```python
from build123d import *

# Parameters (mm, degrees)
SKIZZE19_W = 1.85
SKIZZE19_H = 1
SKIZZE20_W = 1.85
SKIZZE20_H = 1
SKETCH1_W  = 14.101371306
SKETCH1_H  = 11.293421516


with BuildPart() as part:
    # Skizze1 → Rotation1 (revolve)
    with BuildSketch(Plane.XY, mode=Mode.PRIVATE) as rotation1_sk:
        Polygon((180, 19), (180, 0), (-180, 0), (-180, 19), (-79, 19), (-79, 27), (-74, 27), (-74, 19.001), (-44, 19.001), (-44, 19), align=None)
    revolve(rotation1_sk.sketch.rotate(Axis((180, 0, 0), (-1, 0, 0)), 90), axis=Axis((180, 0, 0), (-1, 0, 0)))

    # Skizze19 → Schnitt-Rotation1 (revolve, cut)
    with BuildSketch(Plane.XY, mode=Mode.PRIVATE) as schnitt_rotation1_sk:
        with Locations((171.825, 18.5)):
            Rectangle(SKIZZE19_W, SKIZZE19_H)
    revolve(schnitt_rotation1_sk.sketch.rotate(Axis((-88.99, 0, 0), (1, 0, 0)), 270), axis=Axis((-88.99, 0, 0), (1, 0, 0)), mode=Mode.SUBTRACT)

    # Skizze20 → Schnitt-Rotation2 (revolve, cut)
    with BuildSketch(Plane.XY, mode=Mode.PRIVATE) as schnitt_rotation2_sk:
        with Locations((-171.825, 18.5)):
            Rectangle(SKIZZE20_W, SKIZZE20_H)
    revolve(schnitt_rotation2_sk.sketch.rotate(Axis((-88.99, 0, 0), (1, 0, 0)), 270), axis=Axis((-88.99, 0, 0), (1, 0, 0)), mode=Mode.SUBTRACT)

    # Sketch1 → Cut-Revolve1 (revolve, cut)
    with BuildSketch(Plane.XY, mode=Mode.PRIVATE) as cut_revolve1_sk:
        with Locations((-76.280304753, 24.646710758)):
            Rectangle(SKETCH1_W, SKETCH1_H)
    revolve(cut_revolve1_sk.sketch.rotate(Axis((-191.164691911, 0, 0), (1, 0, 0)), 90), axis=Axis((-191.164691911, 0, 0), (1, 0, 0)), mode=Mode.SUBTRACT)


solid = part.part
```
The listing builds one solid part. Answer for the finished solid, in the listing's coordinates (mm). A direction names the side the tool comes from. Give positions to 0.01 mm unless a question says otherwise; leave off trailing zeros. Order: outer loops, then holes, each group sorted by start corner. A loop starts at its lowest first (then second) coordinate and runs counter-clockwise, first axis right, second up. Notation, with made-up numbers: (-16, 8.5) -> (0, 8.5) arc R21 cw to (0, 37.5) -> close; hole circle Ø6 at (-26.5, -37.75). An arc over 180 degrees is marked (long way). Answer as a JSON object with one key per item and string values. Group by question number.
Item 1: Flat-ended cylindrical pins translate along their axes: pin 1 (3 mm diameter, centred on x = -58, z = 12, fed in from +Y); pin 2 (12 mm diameter, centred on x = 71, z = 3, fed in from -Y); pin 3 (6 mm diameter, centred on x = 109, y = -11, fed in from -Z). Find the tip coordinate at first contact, or state that the pin passes through.
Item 2: Determine the mould class of faces 1 (the flat face through (180, 0, 0)), 2 (the flat face through (-180, 0, 0)), 3 (the flat face through (-170.9, -17, 7)) for opening direction X: pulls with the +X half, pulls with the -X half, needs draft (parallel to the pull), parting line crosses it, or undercut.
Item 3: Consider L1, parallel to X at y = -12.5, z = 13; L2, parallel to Y at x = -81.5, z = -0.5; L3, parallel to Z at x = 116.5, y = -1.5. Determine where each line is inside the solid, lowest interval first. Write a range as from..to.
Item 4: The part is cut by section B-B on x = -102. Write down the section's boundary in (y, z).
Item 5: A tool of negligible diameter and unlimited length cuts with its end or side. For faces 4 (the cylindrical face through (64.954, 18.548, 4.119)), 5 (the flat face through (172.75, -17, 7)), from which of +Z, -Z, +X, -X, +Y, -Y can it reach the whole face along a straight path? Write none if from no direction.
Result set:
{
 "1": {"pin 1": "y = 15.84", "pin 2": "y = -19", "pin 3": "z = -17.23"},
 "2": {"face 1": "pulls with the +X half", "face 2": "pulls with the -X half", "face 3": "undercut"},
 "3": {"L1": "-180..-172.75, -170.9..170.9, 172.75..180", "L2": "-18.99..18.99", "L3": "-18.94..18.94"},
 "4": {"outline": "circle Ø38 at (0, 0)"},
 "5": {"face 4": "+X, -X", "face 5": "none"}
}
